Design review of the part built by this model. Coordinates are the model's own, in mm. A direction names the side the tool comes from. Give positions to 0.01 mm unless a question says otherwise; leave off trailing zeros. Loops run counter-clockwise (first coordinate to the right, second up) from the corner with the lowest first, then second, coordinate; pieces in that order, holes last. Notation, with made-up numbers: M -24.5,37.25 L 19.5,37.25 A17 ccw 19.5,61.25 Z; hole C 35,-12.75 d9. An arc over 180 degrees is marked long. Use a Markdown table: item, result. Add a question column.
(1) Add section C-C, the plane y = 5.5. Give the boundary of the cut face in (x, z) (3 decimals), then the cut area to 3 significant figures.
(2) Add section A-A, the plane z = 8.7. Give the boundary of the cut face in (x, y) (3 decimals).
(3) For probe 1 along X at (y, z) = (0.55, 7.5); probe 2 along Y at (x, z) = (-2.75, -2); probe 3 along X at (y, z) = (1.75, 8.75), list the stretches that pass through material, from the lowest coordinate up.
(4) Insertion check: pin 1 Ø8 at (x, z) = (3.5, -8) entering from +Y; pin 2 Ø4 at (y, z) = (7.5, -4.5) entering from +X (3 decimals); pin 3 Ø1.6 at (y, z) = (2.5, -1.5) entering from +X. Each pin has a flat end and moves straight along its axis. Give the tip position at first contact, or say it passes through.
(5) Add section B-B, the plane x = 5.5. Give the boundary of the cut face in (y, z).
(6) For faces 1 (the face through (-7, 3.5, -9)), 2 (the face through (-2, 1, -10)), 3 (the face through (2, 2, 0)), list the 3-axis set-ups (+Z, -Z, +X, -X, +Y, -Y) from which the entire face can be reached by the end or side of a thin tool; tool diameter is ignored.
(7) Draft analysis for pull direction X (two halves, no side actions). For faces 4 (the face through (-5.1, 2, 1)), 5 (the face through (0, 1, 10)), 6 (the face through (-5.1, 2, 4)), state which applies: pulls with the +X half, pulls with the -X half, needs draft (parallel to the pull), parting line crosses it, or undercut.
(8) Add section D-D, the plane x = 0.5. Give the boundary of the cut face in (y, z).
```python
from build123d import *

# Parameters (mm, degrees)
SKETCH1_W           = 15
SKETCH1_H           = 20
BOSS_EXTRUDE1_DEPTH = 1.5
SKETCH2_R           = 1.5
CUT_EXTRUDE1_DEPTH  = 13.589678312
SKETCH3_W           = 4
SKETCH3_H           = 4
BOSS_EXTRUDE2_DEPTH = 1
FILLET2_R           = 0.5
SKETCH4_W           = 2.4
SKETCH4_H           = 2.4
BOSS_EXTRUDE3_DEPTH = 2
SKETCH5_R           = 0.375
BOSS_EXTRUDE4_DEPTH = 5


with BuildPart() as part:
    # Sketch1 → Boss-Extrude1 (new body)
    with BuildSketch(Plane(origin=(0, 0, 0), x_dir=(1, 0, 0), z_dir=(0, 1, 0))):
        Rectangle(SKETCH1_W, SKETCH1_H)
    extrude(amount=BOSS_EXTRUDE1_DEPTH)

    # Sketch2 → Cut-Extrude1 (cut, through all)
    with BuildSketch(Plane(origin=(0, 1.5, 0), x_dir=(1, 0, 0), z_dir=(0, 1, 0))):
        with Locations(Location((5.5, -7.5, 0), (0, 0, 270))):
            Circle(SKETCH2_R)
        with Locations(Location((5.5, 7.5, 0), (0, 0, 90))):
            Circle(SKETCH2_R)
    extrude(amount=-CUT_EXTRUDE1_DEPTH, mode=Mode.SUBTRACT)

    # Sketch3 → Boss-Extrude2 (add)
    with BuildSketch(Plane(origin=(0, 1.5, 0), x_dir=(1, 0, 0), z_dir=(0, 1, 0))):
        Rectangle(SKETCH3_W, SKETCH3_H)
    extrude(amount=BOSS_EXTRUDE2_DEPTH)

    # Fillet2
    fillet2_edges = [part.edges().sort_by_distance(p)[0] for p in [
        (-2, 2, -2),
        (-2, 2, 2),
        (2, 2, 2),
        (2, 2, -2),
    ]]
    fillet(fillet2_edges, radius=FILLET2_R)

    # Sketch4 → Boss-Extrude3 (add)
    with BuildSketch(Plane(origin=(0, 1.5, 0), x_dir=(1, 0, 0), z_dir=(0, 1, 0))):
        with Locations((-6.3, 8.8)):
            Rectangle(SKETCH4_W, SKETCH4_H)
        with Locations((-6.3, 6.3)):
            Rectangle(SKETCH4_W, SKETCH4_H)
        with Locations((-6.3, 3.8)):
            Rectangle(SKETCH4_W, SKETCH4_H)
        with Locations((-6.3, 1.3)):
            Rectangle(SKETCH4_W, SKETCH4_H)
        with Locations((-6.3, -1.2)):
            Rectangle(SKETCH4_W, SKETCH4_H)
        with Locations((-6.3, -3.7)):
            Rectangle(SKETCH4_W, SKETCH4_H)
        with Locations((-6.3, -6.2)):
            Rectangle(SKETCH4_W, SKETCH4_H)
        with Locations((-6.3, -8.7)):
            Rectangle(SKETCH4_W, SKETCH4_H)
    extrude(amount=BOSS_EXTRUDE3_DEPTH)

    # Sketch5 → Boss-Extrude4 (add)
    with BuildSketch(Plane(origin=(0, 3.5, 0), x_dir=(1, 0, 0), z_dir=(0, 1, 0))):
        with Locations(Location((-6.3, 8.8, 0), (0, 0, 270))):
            Circle(SKETCH5_R)
        with Locations(Location((-6.3, 6.3, 0), (0, 0, 90))):
            Circle(SKETCH5_R)
        with Locations(Location((-6.3, 3.8, 0), (0, 0, 90))):
            Circle(SKETCH5_R)
        with Locations(Location((-6.3, 1.3, 0), (0, 0, 90))):
            Circle(SKETCH5_R)
        with Locations(Location((-6.3, -1.2, 0), (0, 0, 90))):
            Circle(SKETCH5_R)
        with Locations(Location((-6.3, -3.7, 0), (0, 0, 90))):
            Circle(SKETCH5_R)
        with Locations(Location((-6.3, -6.2, 0), (0, 0, 90))):
            Circle(SKETCH5_R)
        with Locations(Location((-6.3, -8.7, 0), (0, 0, 90))):
            Circle(SKETCH5_R)
    extrude(amount=BOSS_EXTRUDE4_DEPTH)


solid = part.part
```
Established:
| question | item | result |
|---|---|---|
| 1 | outline | C -6.3,-8.8 d0.75; C -6.3,-6.3 d0.75; C -6.3,-3.8 d0.75; C -6.3,-1.3 d0.75; C -6.3,1.2 d0.75; C -6.3,3.7 d0.75; C -6.3,6.2 d0.75; C -6.3,8.7 d0.75 |
| 1 | area | 3.53 mm^2 |
| 2 | outline | M -7.5,0 L 4.6,0 L 4.6,1.5 L -5.1,1.5 L -5.1,3.5 L -5.925,3.5 L -5.925,8.5 L -6.675,8.5 L -6.675,3.5 L -7.5,3.5 Z; M 6.4,0 L 7.5,0 L 7.5,1.5 L 6.4,1.5 Z |
| 3 | probe 1 | -7.5 to 4, 7 to 7.5 |
| 3 | probe 2 | 0 to 1.5 |
| 3 | probe 3 | -7.5 to -5.1 |
| 4 | pin 1 | y = 1.5 |
| 4 | pin 2 | x = -5.925 |
| 4 | pin 3 | x = 2 |
| 5 | outline | M 0,-10 L 1.5,-10 L 1.5,-9 L 0,-9 Z; M 0,-6 L 1.5,-6 L 1.5,6 L 0,6 Z; M 0,9 L 1.5,9 L 1.5,10 L 0,10 Z |
| 6 | face 1 | +Y |
| 6 | face 2 | -Z, +X, -X, +Y, -Y |
| 6 | face 3 | +Z, -Z, +X, +Y |
| 7 | face 4 | undercut |
| 7 | face 5 | needs draft |
| 7 | face 6 | pulls with the +X half |
| 8 | outline | M 0,-10 L 1.5,-10 L 1.5,-2 L 2.5,-2 L 2.5,2 L 1.5,2 L 1.5,10 L 0,10 Z |
